```python
from build123d import *

# Parameters (mm, degrees)
BOSS_EXTRUDE1_DEPTH = 5.08
SKETCH2_W           = 12.7
SKETCH2_H           = 5.08
BOSS_EXTRUDE2_DEPTH = 6.35
FILLET3_SIZE        = 6.35
FILLET3_SIZE_2      = 12.7
BOSS_EXTRUDE3_START = -5.08
BOSS_EXTRUDE3_DEPTH = 5.08


with BuildPart() as part:
    # Sketch1 → Boss-Extrude1 (new body)
    with BuildSketch(Plane(origin=(0, 0, 0), x_dir=(1, 0, 0), z_dir=(0, 1, 0))):
        with BuildLine():
            Line((0, 120.65), (12.7, 120.65))
            ThreePointArc((12.7, 120.65), (89.032177029, 89.032177029), (120.65, 12.7))
            Line((120.65, 12.7), (120.65, 0))
            Line((120.65, 0), (107.95, 0))
            Line((107.95, 0), (107.95, 25.4))
            Line((107.95, 25.4), (25.4, 107.95))
            Line((25.4, 107.95), (0, 107.95))
            Line((0, 107.95), (0, 120.65))
        make_face()
        with BuildLine():
            Line((73.363460454, 75.909044866), (79.798132163, 82.343716575))
            ThreePointArc((79.798132163, 82.343716575), (82.343716575, 82.343716575), (82.343716575, 79.798132163))
            Line((82.343716575, 79.798132163), (75.909044866, 73.363460454))
            ThreePointArc((75.909044866, 73.363460454), (73.363460454, 73.363460454), (73.363460454, 75.909044866))
        make_face(mode=Mode.SUBTRACT)
    extrude(amount=BOSS_EXTRUDE1_DEPTH)

    # Sketch2 → Boss-Extrude2 (add)
    with BuildSketch(Plane.ZY):
        with Locations((-114.3, 2.54)):
            Rectangle(SKETCH2_W, SKETCH2_H)
    extrude(amount=BOSS_EXTRUDE2_DEPTH)

    # Fillet3
    # an asymmetric fillet: 12.7, 6.35 mm, written as the material it takes off along each edge
    with BuildSketch(Plane(origin=(-6.35, 36.83, -120.65), x_dir=(1, 0, 0), z_dir=(0, -1, 0))) as fillet3_piece_1:
        with BuildLine():
            Bezier((FILLET3_SIZE, 0), (0, 0), (0, FILLET3_SIZE_2), weights=[1, 0.707106781, 1])
            Line((0, FILLET3_SIZE_2), (0, 0))
            Line((0, 0), (FILLET3_SIZE, 0))
        make_face()
    extrude(amount=68.58, mode=Mode.SUBTRACT)

    # Sketch3 → Boss-Extrude3 (add)
    with BuildSketch(Plane(origin=(0, 5.08, 0), x_dir=(1, 0, 0), z_dir=(0, 1, 0)).offset(BOSS_EXTRUDE3_START)):
        with BuildLine():
            ThreePointArc((12.7, 120.65), (68.239816798, 105.266361331), (107.95, 63.5))
            Line((107.95, 63.5), (107.95, 104.894556371))
            add(Edge.make_bspline(
                [(107.95, 104.894556371), (87.95, 120.65), (12.7, 120.65)],
                knots=[0.5, 0.5, 0.5, 1, 1, 1], degree=2, weights=[1.440625, 1.440625, 1]))
        make_face()
        with BuildLine():
            Line((120.65, 12.7), (120.65, 0))
            ThreePointArc((120.65, 0), (126.049146067, 7.835495184), (127.95, 17.159256086))
            Line((127.95, 17.159256086), (127.95, 29.859256086))
            add(Edge.make_bspline(
                [(127.95, 29.859256086), (127.95, 89.139112741), (107.95, 104.894556371)],
                knots=[0, 0, 0, 0.5, 0.5, 0.5], degree=2, weights=[1, 1.440625, 1.440625]))
            Line((107.95, 104.894556371), (107.95, 63.5))
            ThreePointArc((107.95, 63.5), (117.426882891, 38.881720723), (120.65, 12.7))
        make_face()
        with BuildLine():
            Line((120.65, 0), (107.95, 0))
            Line((107.95, 0), (107.95, -6.35))
            ThreePointArc((107.95, -6.35), (114.784215424, -4.143430847), (120.65, 0))
        make_face()
    extrude(amount=BOSS_EXTRUDE3_DEPTH)


solid = part.part
```
Geometry check sheet. Reference: the model listing, model coordinates, mm. A direction names the side the tool comes from. Give positions to 0.01 mm unless a question says otherwise; leave off trailing zeros. Loops run counter-clockwise (first coordinate to the right, second up) from the corner with the lowest first, then second, coordinate; pieces in that order, holes last. Notation, with made-up numbers: M -27,18.5 L 14,18.5 A23 ccw 14,42.5 Z; hole C 1,85 d9. An arc over 180 degrees is marked long. Write item = value, one per line.
(1) Tool access check on faces 4 (the face through (79.171, 2.504, -76.626)), 5 (the face through (90, 5.08, -72)), 6 (the face through (10, 3, -107.95)). Record the directions out of +Z, -Z, +X, -X, +Y, -Y that give a thin tool (end or side, any length) a straight path to the whole face; none if there is none.
Answer below:
face_4 = +Y, -Y
face_5 = +Z, -Z, +X, -X, +Y
face_6 = +Z, -X, +Y, -Y
(2) Gauge pin test, flat ends, axial feed: pin 1 Ø3 at (y, z) = (2.5, -91) entering from +X; pin 2 Ø1 at (y, z) = (1, -16.5) entering from -X; pin 3 Ø1.5 at (x, y) = (100, 4) entering from +Z. Record the tip position at first contact, or that the pin passes through.
Answer below:
pin_1 = 119.8
pin_2 = 107.95
pin_3 = -32.6
(3) Release check for a two-part mould opening along X. For faces 1 (the face through (107.95, 3, -10)), 2 (the face through (90, 0, -72)), 3 (the face through (76.536, 2.504, -79.081)) record: released by +X, released by -X, zero draft, split by the parting line, or undercut.
Answer below:
face_1 = released by -X
face_2 = zero draft
face_3 = undercut
(4) Sectioned sample at A-A, the plane z = -8.5. Record the cut outline in (x, y).
Answer below:
outline = M 107.95,0 L 126.32,0 L 126.32,5.08 L 107.95,5.08 Z
(5) Material ranges on line 1 (Z direction, x = 12.5, y = 2.45); line 2 (X direction, y = 2.85, z = -16.5), recorded low to high. Write a range as [from, to].
Answer below:
line_1 = [-120.65, -107.95]
line_2 = [107.95, 127.94]
